Can you work these out from the model? Positions are in its coordinate system, mm. Give positions to 0.01 mm unless a question says otherwise; leave off trailing zeros. Loops run counter-clockwise (first coordinate to the right, second up) from the corner with the lowest first, then second, coordinate; pieces in that order, holes last. Notation, with made-up numbers: (73, -16.5) - (104, -16.5) arc R30 ccw to (104, 11.5) - close; hole circle Ø5 at (0.5, 42). An arc over 180 degrees is marked (long way). Write item = value, one per line.
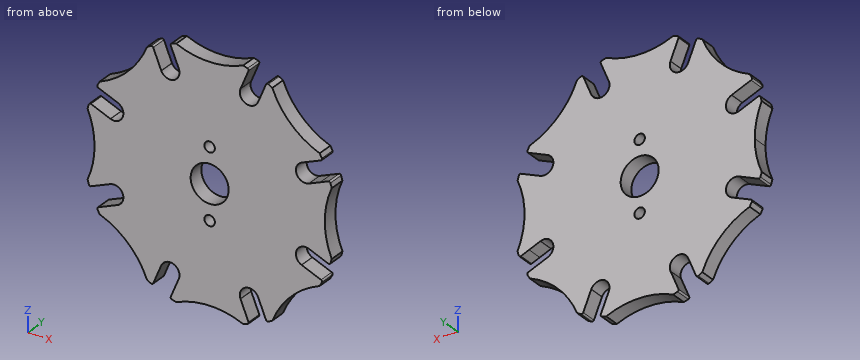
from build123d import *

# Parameters (mm, degrees)
BOSS_EXTRUDE1_DEPTH = 5
SKETCH3_R           = 1.65
SKETCH3_R_2         = 6
CUT_EXTRUDE1_DEPTH  = 10
FILLET2_R           = 0.5


with BuildPart() as part:
    # Sketch2 → Boss-Extrude1 (new body)
    with BuildSketch(Plane(origin=(0, 0, 0), x_dir=(1, 0, 0), z_dir=(0, 1, 0))):
        with BuildLine():
            ThreePointArc((31.282579036, -9.713898359), (32.385596017, -4.912508835), (32.756061614, 0))
            ThreePointArc((32.756061614, 0), (32.385596017, 4.912508835), (31.282579036, 9.713898359))
            ThreePointArc((31.282579036, 9.713898359), (27.491016293, 11.387151792), (28.988887171, 15.251360368))
            ThreePointArc((28.988887171, 15.251360368), (23.162033292, 23.162033292), (15.251360368, 28.988887171))
            ThreePointArc((15.251360368, 28.988887171), (11.387151792, 27.491016293), (9.713898359, 31.282579036))
            ThreePointArc((9.713898359, 31.282579036), (0, 32.756061614), (-9.713898359, 31.282579036))
            ThreePointArc((-9.713898359, 31.282579036), (-11.387151792, 27.491016293), (-15.251360368, 28.988887171))
            ThreePointArc((-15.251360368, 28.988887171), (-23.162033292, 23.162033292), (-28.988887171, 15.251360368))
            ThreePointArc((-28.988887171, 15.251360368), (-27.491016293, 11.387151792), (-31.282579036, 9.713898359))
            ThreePointArc((-31.282579036, 9.713898359), (-32.756061614, 0), (-31.282579036, -9.713898359))
            ThreePointArc((-31.282579036, -9.713898359), (-27.491016293, -11.387151792), (-28.988887171, -15.251360368))
            ThreePointArc((-28.988887171, -15.251360368), (-23.162033292, -23.162033292), (-15.251360368, -28.988887171))
            ThreePointArc((-15.251360368, -28.988887171), (-11.387151792, -27.491016293), (-9.713898359, -31.282579036))
            ThreePointArc((-9.713898359, -31.282579036), (0, -32.756061614), (9.713898359, -31.282579036))
            ThreePointArc((9.713898359, -31.282579036), (11.387151792, -27.491016293), (15.251360368, -28.988887171))
            ThreePointArc((15.251360368, -28.988887171), (23.162033292, -23.162033292), (28.988887171, -15.251360368))
            ThreePointArc((28.988887171, -15.251360368), (27.491016293, -11.387151792), (31.282579036, -9.713898359))
        make_face()
        with BuildLine():
            Line((9.763563492, 31.410705188), (12.492586098, 37.999148577))
            ThreePointArc((12.492586098, 37.999148577), (11.533874506, 38.301040963), (10.567880231, 38.578749428))
            ThreePointArc((10.567880231, 38.578749428), (0, 36.37003279), (-10.567880231, 38.578749428))
            ThreePointArc((-10.567880231, 38.578749428), (-11.533874506, 38.301040963), (-12.492586098, 37.999148577))
            Line((-12.492586098, 37.999148577), (-9.763563492, 31.410705188))
            ThreePointArc((-9.763563492, 31.410705188), (-9.737997226, 31.346926513), (-9.713898359, 31.282579036))
            ThreePointArc((-9.713898359, 31.282579036), (0, 32.756061614), (9.713898359, 31.282579036))
            ThreePointArc((9.713898359, 31.282579036), (9.737997226, 31.346926513), (9.763563492, 31.410705188))
        make_face()
        with BuildLine():
            ThreePointArc((-18.035863293, 35.703047983), (-18.927244915, 35.238606668), (-19.806675556, 34.751915104))
            ThreePointArc((-19.806675556, 34.751915104), (-25.717496818, 25.717496818), (-34.751915104, 19.806675556))
            ThreePointArc((-34.751915104, 19.806675556), (-35.238606668, 18.927244915), (-35.703047983, 18.035863293))
            Line((-35.703047983, 18.035863293), (-29.114604594, 15.306840687))
            ThreePointArc((-29.114604594, 15.306840687), (-29.05142818, 15.279820434), (-28.988887171, 15.251360368))
            ThreePointArc((-28.988887171, 15.251360368), (-23.162033292, 23.162033292), (-15.251360368, 28.988887171))
            ThreePointArc((-15.251360368, 28.988887171), (-15.279820434, 29.05142818), (-15.306840687, 29.114604594))
            Line((-15.306840687, 29.114604594), (-18.035863293, 35.703047983))
        make_face()
        with BuildLine():
            ThreePointArc((-37.999148577, 12.492586098), (-38.301040963, 11.533874506), (-38.578749428, 10.567880231))
            ThreePointArc((-38.578749428, 10.567880231), (-36.928113831, 5.3981136), (-36.37003279, 0))
            ThreePointArc((-36.37003279, 0), (-36.928113831, -5.3981136), (-38.578749428, -10.567880231))
            ThreePointArc((-38.578749428, -10.567880231), (-38.301040963, -11.533874506), (-37.999148577, -12.492586098))
            Line((-37.999148577, -12.492586098), (-31.410705188, -9.763563492))
            ThreePointArc((-31.410705188, -9.763563492), (-31.346926513, -9.737997226), (-31.282579036, -9.713898359))
            ThreePointArc((-31.282579036, -9.713898359), (-32.756061614, 0), (-31.282579036, 9.713898359))
            ThreePointArc((-31.282579036, 9.713898359), (-31.346926513, 9.737997226), (-31.410705188, 9.763563492))
            Line((-31.410705188, 9.763563492), (-37.999148577, 12.492586098))
        make_face()
        with BuildLine():
            ThreePointArc((-15.306840687, -29.114604594), (-15.279820434, -29.05142818), (-15.251360368, -28.988887171))
            ThreePointArc((-15.251360368, -28.988887171), (-23.162033292, -23.162033292), (-28.988887171, -15.251360368))
            ThreePointArc((-28.988887171, -15.251360368), (-29.05142818, -15.279820434), (-29.114604594, -15.306840687))
            Line((-29.114604594, -15.306840687), (-35.703047983, -18.035863293))
            ThreePointArc((-35.703047983, -18.035863293), (-35.238606668, -18.927244915), (-34.751915104, -19.806675556))
            ThreePointArc((-34.751915104, -19.806675556), (-25.717496818, -25.717496818), (-19.806675556, -34.751915104))
            ThreePointArc((-19.806675556, -34.751915104), (-18.927244915, -35.238606668), (-18.035863293, -35.703047983))
            Line((-18.035863293, -35.703047983), (-15.306840687, -29.114604594))
        make_face()
        with BuildLine():
            ThreePointArc((9.763563492, -31.410705188), (9.737997226, -31.346926513), (9.713898359, -31.282579036))
            ThreePointArc((9.713898359, -31.282579036), (0, -32.756061614), (-9.713898359, -31.282579036))
            ThreePointArc((-9.713898359, -31.282579036), (-9.737997226, -31.346926513), (-9.763563492, -31.410705188))
            Line((-9.763563492, -31.410705188), (-12.492586098, -37.999148577))
            ThreePointArc((-12.492586098, -37.999148577), (-11.533874506, -38.301040963), (-10.567880231, -38.578749428))
            ThreePointArc((-10.567880231, -38.578749428), (0, -36.37003279), (10.567880231, -38.578749428))
            ThreePointArc((10.567880231, -38.578749428), (11.533874506, -38.301040963), (12.492586098, -37.999148577))
            Line((12.492586098, -37.999148577), (9.763563492, -31.410705188))
        make_face()
        with BuildLine():
            ThreePointArc((29.114604594, -15.306840687), (29.05142818, -15.279820434), (28.988887171, -15.251360368))
            ThreePointArc((28.988887171, -15.251360368), (23.162033292, -23.162033292), (15.251360368, -28.988887171))
            ThreePointArc((15.251360368, -28.988887171), (15.279820434, -29.05142818), (15.306840687, -29.114604594))
            Line((15.306840687, -29.114604594), (18.035863293, -35.703047983))
            ThreePointArc((18.035863293, -35.703047983), (18.927244915, -35.238606668), (19.806675556, -34.751915104))
            ThreePointArc((19.806675556, -34.751915104), (25.717496818, -25.717496818), (34.751915104, -19.806675556))
            ThreePointArc((34.751915104, -19.806675556), (35.238606668, -18.927244915), (35.703047983, -18.035863293))
            Line((35.703047983, -18.035863293), (29.114604594, -15.306840687))
        make_face()
        with BuildLine():
            ThreePointArc((34.934473466, -11.223156103), (33.305699609, -5.716308055), (32.756061614, 0))
            ThreePointArc((32.756061614, 0), (32.385596017, -4.912508835), (31.282579036, -9.713898359))
            ThreePointArc((31.282579036, -9.713898359), (31.346926513, -9.737997226), (31.410705188, -9.763563492))
            Line((31.410705188, -9.763563492), (34.934473466, -11.223156103))
        make_face()
        with BuildLine():
            ThreePointArc((38.578749428, 10.567880231), (38.301040963, 11.533874506), (37.999148577, 12.492586098))
            Line((37.999148577, 12.492586098), (34.934473466, 11.223156103))
            ThreePointArc((34.934473466, 11.223156103), (33.305699609, 5.716308055), (32.756061614, 0))
            ThreePointArc((32.756061614, 0), (33.305699609, -5.716308055), (34.934473466, -11.223156103))
            Line((34.934473466, -11.223156103), (37.999148577, -12.492586098))
            ThreePointArc((37.999148577, -12.492586098), (38.301040963, -11.533874506), (38.578749428, -10.567880231))
            ThreePointArc((38.578749428, -10.567880231), (36.37003279, 0), (38.578749428, 10.567880231))
        make_face()
        with BuildLine():
            ThreePointArc((32.756061614, 0), (33.305699609, 5.716308055), (34.934473466, 11.223156103))
            Line((34.934473466, 11.223156103), (31.410705188, 9.763563492))
            ThreePointArc((31.410705188, 9.763563492), (31.346926513, 9.737997226), (31.282579036, 9.713898359))
            ThreePointArc((31.282579036, 9.713898359), (32.385596017, 4.912508835), (32.756061614, 0))
        make_face()
        with BuildLine():
            Line((29.114604594, 15.306840687), (35.703047983, 18.035863293))
            ThreePointArc((35.703047983, 18.035863293), (35.238606668, 18.927244915), (34.751915104, 19.806675556))
            ThreePointArc((34.751915104, 19.806675556), (25.717496818, 25.717496818), (19.806675556, 34.751915104))
            ThreePointArc((19.806675556, 34.751915104), (18.927244915, 35.238606668), (18.035863293, 35.703047983))
            Line((18.035863293, 35.703047983), (15.306840687, 29.114604594))
            ThreePointArc((15.306840687, 29.114604594), (15.279820434, 29.05142818), (15.251360368, 28.988887171))
            ThreePointArc((15.251360368, 28.988887171), (23.162033292, 23.162033292), (28.988887171, 15.251360368))
            ThreePointArc((28.988887171, 15.251360368), (29.05142818, 15.279820434), (29.114604594, 15.306840687))
        make_face()
    extrude(amount=BOSS_EXTRUDE1_DEPTH)

    # Sketch3 → Cut-Extrude1 (cut)
    with BuildSketch(Plane(origin=(0, 5, 0), x_dir=(1, 0, 0), z_dir=(0, 1, 0))):
        with Locations(Location((0, 11, 0), (0, 0, 270))):
            Circle(SKETCH3_R)
        with Locations(Location((0, 0, 0), (0, 0, 270))):
            Circle(SKETCH3_R_2)
        with Locations(Location((0, -11, 0), (0, 0, 270))):
            Circle(SKETCH3_R)
    extrude(amount=-CUT_EXTRUDE1_DEPTH, mode=Mode.SUBTRACT)

    # Fillet2
    fillet2_edges = [part.edges().sort_by_distance(p)[0] for p in [
        (18.035863293, 2.5, -35.703047983),
        (35.703047983, 2.5, -18.035863293),
        (37.999148577, 2.5, -12.492586098),
        (37.999148577, 2.5, 12.492586098),
        (35.703047983, 2.5, 18.035863293),
        (18.035863293, 2.5, 35.703047983),
        (12.492586098, 2.5, 37.999148577),
        (-12.492586098, 2.5, 37.999148577),
        (-18.035863293, 2.5, 35.703047983),
        (-35.703047983, 2.5, 18.035863293),
        (-37.999148577, 2.5, 12.492586098),
        (-37.999148577, 2.5, -12.492586098),
        (-35.703047983, 2.5, -18.035863293),
        (-18.035863293, 2.5, -35.703047983),
        (-12.492586098, 2.5, -37.999148577),
        (12.492586098, 2.5, -37.999148577),
    ]]
    fillet(fillet2_edges, radius=FILLET2_R)


solid = part.part
Q1. I need wall thicknesses on L1, parallel to X at y = 3.35, z = -11; L2, parallel to Z at x = 10, y = 1.15; L3, parallel to Z at x = -1, y = 1.2. Which ranges of each line are inside material? Lowest first, please.
Output:
L1 = -38.46 to -34.4, -27.69 to -1.65, 1.65 to 27.69, 34.4 to 38.46
L2 = -38.34 to -31.98, -28.66 to 28.66, 31.98 to 38.34
L3 = -36.39 to -12.31, -9.69 to -5.92, 5.92 to 9.69, 12.31 to 36.39
Q2. For pin 1 (1 mm diameter, centred on x = 9.5, y = 4, fed in from -Z), with a flat end and sliding along its axis, tell me the tip position at first contact or that it passes through.
Output:
pin_1 = -38.34
Q3. Imagine slicing it at C-C, the plane z = 25. Write out the boundary of the cut face in (x, y), then the cut area to 3 significant figures.
Output:
outline = (-26.46, 0) - (26.46, 0) - (26.46, 5) - (-26.46, 5) - close
area = 265 mm2
Q4. Imagine slicing it at A-A, the plane x = 0. Write out the boundary of the cut face in (y, z), then the cut area to 3 significant figures.
Output:
outline = (0, -36.37) - (5, -36.37) - (5, -12.65) - (0, -12.65) - close; (0, -9.35) - (5, -9.35) - (5, -6) - (0, -6) - close; (0, 6) - (5, 6) - (5, 9.35) - (0, 9.35) - close; (0, 12.65) - (5, 12.65) - (5, 36.37) - (0, 36.37) - close
area = 271 mm2
Q5. Imagine slicing it at B-B, the plane y = 3. Give the number of separate pieces and of enclosed holes in the cut face, then the cut area to 3 significant figures.
Output:
separate_pieces = 1
enclosed_holes = 3
area = 4,020 mm2
Q6. Imagine slicing it at D-D, the plane z = 7.5. Write out the boundary of the cut face in (x, y), then the cut area to 3 significant figures.
Output:
outline = (-37.46, 0) - (37.46, 0) - (37.46, 5) - (-37.46, 5) - close
area = 375 mm2
